from build123d import *

# Parameters (mm, degrees)
SKETCH1_R           = 7.5
SKETCH1_R_2         = 10
BOSS_EXTRUDE1_DEPTH = 10


with BuildPart() as part:
    # Sketch1 → Boss-Extrude1 (new body, symmetric)
    with BuildSketch(Plane.XY):
        with BuildLine():
            Line((0, 0), (87, 0))
            Line((87, 0), (87, 14))
            ThreePointArc((87, 14), (95, 22), (103, 14))
            Line((103, 14), (103, 0))
            Line((103, 0), (130, 0))
            Line((130, 0), (130, 12))
            Line((130, 12), (120, 12))
            ThreePointArc((120, 12), (116.464466094, 13.464466094), (115, 17))
            Line((115, 17), (115, 42))
            ThreePointArc((115, 42), (95, 62), (75, 42))
            ThreePointArc((75, 42), (63.985563365, 27.57012052), (45.874646321, 26.331605267))
            ThreePointArc((45.874646321, 26.331605267), (29.43761269, 29.930536508), (20, 16))
            ThreePointArc((20, 16), (18.340800225, 13.188309736), (15.3, 12))
            Line((15.3, 12), (0, 12))
            Line((0, 12), (0, 0))
        make_face()
        with Locations((35, 16)):
            Circle(SKETCH1_R, mode=Mode.SUBTRACT)
        with Locations((95, 42)):
            Circle(SKETCH1_R_2, mode=Mode.SUBTRACT)
    extrude(amount=BOSS_EXTRUDE1_DEPTH, both=True)


solid = part.part
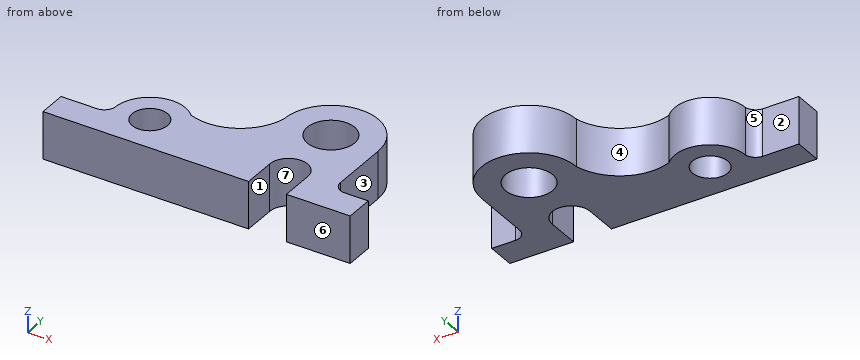
The listing builds one solid part. Answer for the finished solid, in the listing's coordinates (mm). Face numbers are marked on the shaded views. A direction names the side the tool comes from. Give positions to 0.01 mm unless a question says otherwise; leave off trailing zeros. Write each loop counter-clockwise with the first axis right and the second up, starting at its lowest first coordinate (ties: lowest second). Pieces come first, ordered by that corner, then holes.
Item 1: Determine the mould class of the marked faces 5, 6 and 7 for opening direction X: released by +X, released by -X, zero draft, split by the parting line, or undercut.
Item 2: Section C-C, the plane z = -4.5 is taken. Write down the section's boundary in (x, y), plus the area to 3 significant figures.
Item 3: Section A-A, the plane x = 95 is taken. Write down the section's boundary in (y, z), plus the area to 3 significant figures.
Item 4: Section D-D, the plane x = 66 is taken. Write down the section's boundary in (y, z), plus the area to 3 significant figures.
Item 5: Which of the six approach directions +Z, -Z, +X, -X, +Y, -Y give full straight-line access (tool end or side, diameter ignored) to the marked faces 1, 2, 3 and 4?
Item 6: Find the intervals of material crossed by line 1 along Y through (x, z) = (95, -0.5); line 2 along Y through (x, z) = (35, 0.75); line 3 along Y through (x, z) = (122, 7.75), in increasing order.
Item 7: Section B-B, the plane y = 5.5 is taken. Write down the section's boundary in (x, z), plus the area to 3 significant figures.
Item 8: Flat-ended cylindrical pins translate along their axes: P1, Ø6, axis at y = 24.5, z = -3, coming from the +X side; P2, Ø8, axis at x = 123, z = -2.5, coming from the +Y side; P3, Ø12, axis at x = 42.5, z = 0.5, coming from the +Y side. Find the tip coordinate at first contact, or state that the pin passes through.
Completed:
1. face 5: released by -X
1. face 6: zero draft
1. face 7: undercut
2. outline: (0, 0) - (87, 0) - (87, 14) arc R8 cw to (103, 14) - (103, 0) - (130, 0) - (130, 12) - (120, 12) arc R5 cw to (115, 17) - (115, 42) arc R20 ccw to (75, 42) arc R22 cw to (45.87, 26.33) arc R15 ccw to (20, 16) arc R5 cw to (15.3, 12) - (0, 12) - close; hole circle Ø15 at (35, 16); hole circle Ø20 at (95, 42)
2. area: 3,480 mm2
3. outline: (22, -10) - (32, -10) - (32, 10) - (22, 10) - close; (52, -10) - (62, -10) - (62, 10) - (52, 10) - close
3. area: 400 mm2
4. outline: (0, -10) - (28.8, -10) - (28.8, 10) - (0, 10) - close
4. area: 576 mm2
5. face 1: +Z, -Z, -Y
5. face 2: +Z, -Z, -X, +Y
5. face 3: +Z, -Z, +X, +Y
5. face 4: +Z, -Z, +Y
6. line 1: y = 22 to 32, 52 to 62
6. line 2: y = 0 to 8.5, 23.5 to 31
6. line 3: y = 0 to 12
7. outline: (0, -10) - (87, -10) - (87, 10) - (0, 10) - close; (103, -10) - (130, -10) - (130, 10) - (103, 10) - close
7. area: 2,280 mm2
8. P1: stops at x = 115
8. P2: stops at y = 12.1
8. P3: stops at y = 30.92
